from build123d import *

# Parameters (mm, degrees)
SKETCH_1_W           = 90
SKETCH_1_H           = 52
EXTRUDE_1_DEPTH      = 40
SKETCH_2_R           = 6
CUT_EXTRUDE_1_DEPTH  = 66.582009728
SKETCH_3_R           = 1.5
CUT_EXTRUDE_2_DEPTH  = 80.555012413
SKETCH_6_R           = 1.5
CUT_EXTRUDE_4_DEPTH  = 8
SKETCH_8_W           = 17
SKETCH_8_H           = 20
CUT_EXTRUDE_5_DEPTH  = 66.582009728
SKETCH_17_W          = 30
SKETCH_17_H          = 30
CUT_EXTRUDE_18_DEPTH = 38
SKETCH_9_R           = 15.5
CUT_EXTRUDE_17_DEPTH = 30
SKETCH_21_W          = 17
SKETCH_21_H          = 6
EXTRUDE_7_DEPTH      = 40
FILLET_3_R           = 3
CUT_EXTRUDE_START    = -8
SKETCH_24_R          = 1.5
CUT_EXTRUDE_16_DEPTH = 8


with BuildPart() as part:
    # 草圖1 → 填料-伸長1 (new body)
    with BuildSketch(Plane.XY):
        Rectangle(SKETCH_1_W, SKETCH_1_H)
    extrude(amount=EXTRUDE_1_DEPTH)

    # 草圖2 → 除料-伸長1 (cut, through all)
    with BuildSketch(Plane(origin=(0, 0, 0), x_dir=(-1, 0, 0), z_dir=(0, 0, -1))):
        with Locations((-31, -18)):
            Circle(SKETCH_2_R)
        with Locations(Location((35, -18, 0), (0, 0, 180))):
            Circle(SKETCH_2_R)
        with Locations((35, 18)):
            Circle(SKETCH_2_R)
        with Locations(Location((-31, 18, 0), (0, 0, 180))):
            Circle(SKETCH_2_R)
    extrude(amount=-CUT_EXTRUDE_1_DEPTH, mode=Mode.SUBTRACT)

    # 草圖3 → 除料-伸長2 (cut, through all)
    with BuildSketch(Plane(origin=(0, 26, 0), x_dir=(1, 0, 0), z_dir=(0, 1, 0))):
        with Locations(Location((6, -28.8, 0), (0, 0, 270))):
            Circle(SKETCH_3_R)
        with Locations(Location((6, -11.2, 0), (0, 0, 270))):
            Circle(SKETCH_3_R)
        Polygon((3.706406461, -27), (0.242304845, -21), (-6.685898385, -21), (-10.15, -27), (-6.685898385, -33), (0.242304845, -33), align=None)
        Polygon((0.242304845, -7), (3.706406461, -13), (0.242304845, -19), (-6.685898385, -19), (-10.15, -13), (-6.685898385, -7), align=None)
    extrude(amount=-CUT_EXTRUDE_2_DEPTH, mode=Mode.SUBTRACT)

    # 草圖6 → 除料-伸長4 (cut)
    with BuildSketch(Plane(origin=(0, 0, 0), x_dir=(-1, 0, 0), z_dir=(0, 0, -1))):
        with Locations((-19, 15.5)):
            Circle(SKETCH_6_R)
        with Locations((19, 15.5)):
            Circle(SKETCH_6_R)
    extrude(amount=-CUT_EXTRUDE_4_DEPTH, mode=Mode.SUBTRACT)

    # 草圖8 → 除料-伸長5 (cut, through all)
    with BuildSketch(Plane(origin=(0, 0, 0), x_dir=(-1, 0, 0), z_dir=(0, 0, -1))):
        with Locations((36.5, 0)):
            Rectangle(SKETCH_8_W, SKETCH_8_H)
    extrude(amount=-CUT_EXTRUDE_5_DEPTH, mode=Mode.SUBTRACT)

    # 草圖17 → 除料-伸長18 (cut)
    with BuildSketch(Plane.XZ.offset(26)):
        with Locations((0, 20)):
            Rectangle(SKETCH_17_W, SKETCH_17_H)
    extrude(amount=-CUT_EXTRUDE_18_DEPTH, mode=Mode.SUBTRACT)

    # 草圖9 → 除料-伸長17 (cut)
    with BuildSketch(Plane(origin=(45, 0, 0), x_dir=(0, 0, -1), z_dir=(1, 0, 0))):
        with Locations((-20, -3)):
            Circle(SKETCH_9_R)
    extrude(amount=-CUT_EXTRUDE_17_DEPTH, mode=Mode.SUBTRACT)

    # 草圖21 → 填料-伸長7 (add)
    with BuildSketch(Plane.XY.offset(40)):
        with Locations((-36.5, 0)):
            Rectangle(SKETCH_21_W, SKETCH_21_H)
    extrude(amount=-EXTRUDE_7_DEPTH)

    # 圓角3
    fillet_3_edges = [part.edges().sort_by_distance(p)[0] for p in [
        (45, 0, 40),
        (-45, 0, 40),
        (-45, 0, 0),
        (-45, 18, 40),
        (45, 0, 0),
        (-45, 18, 0),
        (-45, -18, 0),
        (-45, -18, 40),
    ]]
    fillet(fillet_3_edges, radius=FILLET_3_R)

    # 草圖24 → 除料-伸長16 (cut)
    with BuildSketch(Plane.XY.offset(40).offset(CUT_EXTRUDE_START)):
        with Locations(Location((-19, 15.5, 0), (0, 0, 180))):
            Circle(SKETCH_24_R)
        with Locations(Location((19, 15.5, 0), (0, 0, 180))):
            Circle(SKETCH_24_R)
    extrude(amount=CUT_EXTRUDE_16_DEPTH, mode=Mode.SUBTRACT)


solid = part.part
Build history of the part. All positions in model axes, mm. A direction names the side the tool comes from. Give positions to 0.01 mm unless a question says otherwise; leave off trailing zeros. Order: outer loops, then holes, each group sorted by start corner. A loop starts at its lowest first (then second) coordinate and runs counter-clockwise, first axis right, second up. Notation, with made-up numbers: M 88,38 L 125,38 A31 cw 125,65 Z; hole C 6,-20.5 d6. An arc over 180 degrees is marked long. Use one line per item in the form item = value.
Q1. Which spindle directions (+Z, -Z, +X, -X, +Y, -Y) get a long thin tool onto all of the face, cutting with end or side? Do faces 1 (the flat face through (15, 9, 32)), 2 (the flat face through (-19, 16, 8)), 3 (the flat face through (-36, 10, 20)), 4 (the flat face through (19, 15, 32)). Say none if no direction does.
Conclusion:
face_1 = -Y
face_2 = -Z
face_3 = +Z, -Z, -X
face_4 = +Z
Q2. Pin check, flat tips, straight feed: P1, Ø3.5, axis at x = -19, y = 15.5, coming from the +Z side; P2, Ø1.5, axis at x = 18.5, y = 16, coming from the +Z side; P3, Ø9, axis at x = -6, z = 18, coming from the -Y side; P4, Ø9, axis at y = -8.5, z = 26.5, coming from the +X side. Stop position of each tip, or through.
Conclusion:
P1 = 40
P2 = 32
P3 = 12
P4 = -15
Q3. Wall check: probe 1 along X at (y, z) = (18.5, 3); probe 2 along Y at (x, z) = (-35, 23); probe 3 along Z at (x, y) = (-7.5, 4). Give the ranges that are in metal, low to high.
Conclusion:
probe_1 = -45 to -40.98, -29.02 to 25.02, 36.98 to 45
probe_2 = -26 to -24, -12 to -10, -3 to 3, 10 to 12, 24 to 26
probe_3 = 0 to 5, 35 to 40
Q4. Slice it at D-D, the plane x = 19. Write the cut outline in (y, z).
Conclusion:
outline = M -26,0 L 14,0 L 14,8 L 17,8 L 17,0 L 26,0 L 26,40 L 17,40 L 17,32 L 14,32 L 14,40 L -26,40 Z; hole C -3,20 d31
Q5. Pull direction Y, two halves, no side cores. Call faces 5 (the cylindrical face through (20.5, 15.43, 35.94)), 6 (the flat face through (-8.44, 19.1, 10.04)): released by +Y, released by -Y, zero draft, split by the parting line, or undercut.
Conclusion:
face_5 = undercut
face_6 = zero draft
Q6. Slice it at B-B, the plane y = 18. State how many separate pieces and enclosed holes the cut face has, and give its area (3 significant figures).
Conclusion:
separate_pieces = 3
enclosed_holes = 4
area = 2,370 mm2
Q7. Slice it at A-A, the plane x = 6. Write the cut outline in (y, z), and give its area (3 significant figures).
Conclusion:
outline = M -26,0 L 26,0 L 26,9.7 L 12,9.7 L 12,5 L -26,5 Z; M -26,35 L 12,35 L 12,30.3 L 26,30.3 L 26,40 L -26,40 Z; M 12,12.7 L 26,12.7 L 26,27.3 L 12,27.3 Z
area = 856 mm2
